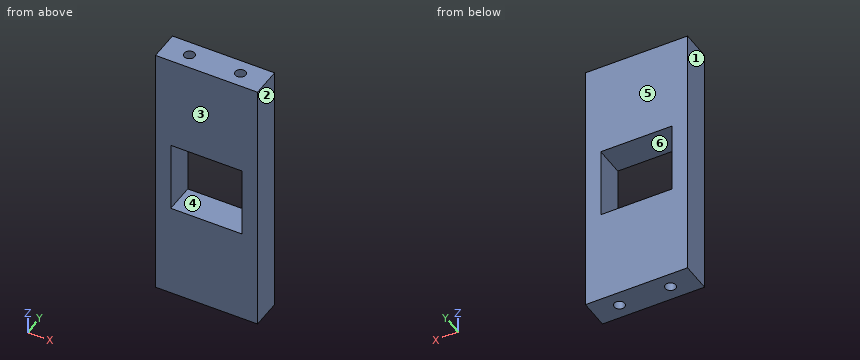
Autodesk Fusion 360 part; units mm, degrees
sketch "Sketch1" plane through (0, 0, 0) normal (0, 1, 0) x (1, 0, 0)
  line L0 (0, 0) -> (20, 0)
  line L1 (20, 0) -> (20, -51.54)
  line L2 (20, -51.54) -> (0, -51.54)
  line L3 (0, -51.54) -> (0, 0)
  dimension "d1" = 20
  dimension "d2" = 51.54
extrude "Extrude1" add sketch "Sketch1" along normal blind 5.92
sketch "Sketch2" plane through (0, 5.92, 0) normal (0, 1, 0) x (-1, 0, 0)
  line L0 (0, 51.54) -> (-20, 51.54)
  line L1 (-20, 51.54) -> (-20, 0)
  line L2 (-20, 0) -> (0, 0)
  line L3 (0, 0) -> (0, 51.54)
  line L4 (-10, 0) -> (-10, 49) construction
  line L5 (0, 25.77) -> (-20, 25.77) construction
  line L6 (-3, 32.77) -> (-17, 32.77)
  line L7 (-17, 32.77) -> (-17, 18.77)
  line L8 (-17, 18.77) -> (-3, 18.77)
  line L9 (-3, 18.77) -> (-3, 32.77)
  line L10 (-3, 32.77) -> (-17, 18.77) construction
  line L11 (-17, 32.77) -> (-3, 18.77) construction
  point P0 (-10, 25.77)
  dimension "d5" = 14
  dimension "d6" = 14
extrude "Extrude2" cut sketch "Sketch2" along normal through all and the other way through all contours L6 L7 L8 L9
sketch "Sketch3" plane through (0, 0, 51.54) normal (0, 0, 1) x (1, 0, 0)
  line L0 (0, 0) -> (20, 0)
  line L1 (20, 0) -> (20, 5.92)
  line L2 (20, 5.92) -> (0, 5.92)
  line L3 (0, 5.92) -> (0, 0)
  line L4 (10, 5.92) -> (10, 0) construction
  line L5 (20, 2.96) -> (0, 2.96) construction
  point P0 (5, 2.96)
  point P1 (15, 2.96)
  dimension "d12" = 10
  dimension "d13" = 5
hole "Hole1" at (5, 2.96, 51.54) direction (0, 0, -1) diameter 2.05 depth 10 tip angle 118
hole "Hole2" at (15, 2.96, 51.54) direction (0, 0, -1) diameter 2.05 depth 10 tip angle 118
sketch "Sketch4" plane through (0, 0, 0) normal (0, 0, -1) x (-1, 0, 0)
  line L0 (-20, 0) -> (0, 0)
  line L1 (0, 0) -> (0, 5.92)
  line L2 (0, 5.92) -> (-20, 5.92)
  line L3 (-20, 5.92) -> (-20, 0)
  line L4 (-20, 2.96) -> (0, 2.96) construction
  point P0 (-15, 2.96)
  point P1 (-5, 2.96)
  dimension "d30" = 10
  dimension "d31" = 5
hole "Hole5" at (15, 2.96, 0) direction (0, 0, 1) diameter 2.05 depth 10 tip angle 118
hole "Hole6" at (5, 2.96, 0) direction (0, 0, 1) diameter 2.05 depth 10 tip angle 118
The model under review builds one solid part; all positions refer to its coordinate system, in mm. Face numbers are marked on the shaded views. A direction names the side the tool comes from. Give positions to 0.01 mm unless a question says otherwise; leave off trailing zeros. Loops run counter-clockwise (first coordinate to the right, second up) from the corner with the lowest first, then second, coordinate; pieces in that order, holes last. Notation, with made-up numbers: (63.25, 59.25) -> (106.25, 59.25) arc R29 ccw to (106.25, 87.25) -> close; hole circle Ø7 at (47.5, 76.5). An arc over 180 degrees is marked (long way). Use CSV: the item, a comma, the result in double quotes.
1. Consider section B-B, the plane z = 24. Write out the cut boundary in (x, y).
Result:
outline,"(0, 0) -> (3, 0) -> (3, 5.92) -> (0, 5.92) -> close; (17, 0) -> (20, 0) -> (20, 5.92) -> (17, 5.92) -> close"
2. The part is to be moulded in two halves that separate along X. For the marked faces 1, 2, 3 and 4, say which applies: +X half, -X half, draft (parallel to the pull), parting line (faces both ways), or undercut.
Result:
face 1,"-X half"
face 2,"+X half"
face 3,"draft"
face 4,"undercut"
3. To check wall thickness, follow probe 1 along X at (y, z) = (2.96, 6.5) (3 decimals); probe 2 along Z at (x, y) = (15.75, 1.7); probe 3 along Y at (x, z) = (5, 47.5) (3 decimals). State the ranges of each line that lie inside material, in increasing order. Write a range as from..to.
Result:
probe 1,"x = 0..3.975, 6.025..13.975, 16.025..20"
probe 2,"z = 0..18.77, 32.77..51.54"
probe 3,"y = 0..1.935, 3.985..5.92"
4. Consider section A-A, the plane x = 12.5. Write out the cut boundary in (y, z), then the cut area to 3 significant figures.
Result:
outline,"(0, 0) -> (5.92, 0) -> (5.92, 18.77) -> (0, 18.77) -> close; (0, 32.77) -> (5.92, 32.77) -> (5.92, 51.54) -> (0, 51.54) -> close"
area,"222 mm²"
5. Machinability: for the marked faces 5 and 6, which of the approach directions +Z, -Z, +X, -X, +Y, -Y give a long, thin tool a straight path to every point of the face, cutting with its end or side? Answer none if there is none.
Result:
face 5,"+Z, -Z, +X, -X, +Y"
face 6,"+Y, -Y"
6. For P1, Ø3, axis at y = 4.5, z = 42.5, coming from the -X side; P2, Ø1.6, axis at x = 5, y = 2.96, coming from the -Z side; P3, Ø1.2, axis at x = 15, y = 2.96, coming from the -Z side, all flat-tipped, find the tip position at first contact; note any pin that passes through.
Result:
P1,"stops at x = 0"
P2,"stops at z = 10.14"
P3,"stops at z = 10.26"
7. Consider section C-C, the plane y = 1.15. Write out the cut boundary in (x, z), then the cut area to 3 significant figures.
Result:
outline,"(0, 0) -> (20, 0) -> (20, 51.54) -> (0, 51.54) -> close; hole (3, 18.77) -> (17, 18.77) -> (17, 32.77) -> (3, 32.77) -> close"
area,"835 mm²"
